The listing builds one solid part. Answer for the finished solid, in the listing's coordinates (mm). A direction names the side the tool comes from. Give positions to 0.01 mm unless a question says otherwise; leave off trailing zeros. Write each loop counter-clockwise with the first axis right and the second up, starting at its lowest first coordinate (ties: lowest second). Pieces come first, ordered by that corner, then holes. Notation, with made-up numbers: (42, 23.5) -> (69, 23.5) arc R18 cw to (69, 49.5) -> close; hole circle Ø3 at (3.5, -33.5). An arc over 180 degrees is marked (long way). One line per question, with ' | ' between items.
Autodesk Inventor part; units mm, degrees
ref_plane "YZ Plane" through (0, 0, 0) normal (1, 0, 0) x (0, 1, 0)
ref_plane "XZ Plane" through (0, 0, 0) normal (0, 1, 0) x (-1, 0, 0)
ref_plane "XY Plane" through (0, 0, 0) normal (0, 0, 1) x (1, 0, 0)
sketch "Esquisse1" plane through (0, 0, 0) normal (0, 1, 0) x (-1, 0, 0)
  line L0 (0, 0) -> (36, 0) construction
  line L1 (36, 0) -> (36, 8) construction
  line L2 (0, 0) -> (0, 13.5) construction
  line L3 (0, 13.5) -> (6.5, 13.5) construction
  line L4 (6.5, 13.5) -> (14.5, 13.5) construction
  line L5 (14.5, 13.5) -> (22.5, 13.5) construction
  line L6 (22.5, 13.5) -> (30.5, 13.5) construction
  circle A0 centre (6.5, 13.5) radius 1
  circle A1 centre (14.5, 13.5) radius 1
  circle A2 centre (22.5, 13.5) radius 1
  circle A3 centre (30.5, 13.5) radius 1
  circle A4 centre (36, 8) radius 1
  circle A5 centre (6.5, -13.5) radius 1
  circle A6 centre (14.5, -13.5) radius 1
  circle A7 centre (22.5, -13.5) radius 1
  circle A8 centre (30.5, -13.5) radius 1
  circle A9 centre (36, -8) radius 1
  line L7 (6.5, 13.5) -> (6.5, 18.5) construction
  line L8 (36, 8) -> (41, 8) construction
  circle A10 centre (0, 0) radius 12 construction
  line L9 (0, 18.5) -> (41, 18.5)
  line L10 (41, 18.5) -> (41, -18.5)
  line L11 (41, -18.5) -> (0, -18.5)
  line L12 (6.5, -13.5) -> (6.5, -18.5) construction
  line L13 (0, 18.5) -> (0, 12)
  line L14 (0, 0) -> (0, -18.5) construction
  line L15 (0, -12) -> (0, -18.5)
  arc A11 (0, -12) -> (0, 12) centre (0, 0) ccw
  dimension "d23" = 36
  dimension "d24" = 8
  dimension "d25" = 13.5
  dimension "d26" = 6.5
  dimension "d27" = 8
  dimension "d28" = 8
  dimension "d29" = 8
  dimension "d30" = 2
  dimension "d31" = 5
  dimension "d33" = 24
extrude "Extrusion2" add sketch "Esquisse1" along normal blind 2
fillet "Congé1" radius 2 1 edges at (0, 1, 12)
fillet "Congé2" radius 2 1 edges at (0, 1, -12)
properties part number "AX12_gabarit"
Item 1: Consider line 1 (Z direction, x = -22.5, y = 0.85); line 2 (Z direction, x = -6.5, y = 1.3); line 3 (X direction, y = 1.45, z = -13). Determine where each line is inside the solid, lowest interval first. Write a range as [from, to].
Answers below:
line 1: [-18.5, -14.5], [-12.5, 12.5], [14.5, 18.5] | line 2: [-18.5, -14.5], [-12.5, -10.09], [10.09, 12.5], [14.5, 18.5] | line 3: [-41, -31.37], [-29.63, -23.37], [-21.63, -15.37], [-13.63, -7.37], [-5.63, -0.19]
Item 2: Determine the mould class of faces 3 (the face through (-0.501, 1.014, -12.532)), 4 (the face through (-41, 1, 0)), 5 (the face through (-20, 1, 18.5)) for opening direction Z: pulls with the +Z half, pulls with the -Z half, needs draft (parallel to the pull), parting line crosses it, or undercut.
Answers below:
face 3: undercut | face 4: needs draft | face 5: pulls with the +Z half
Item 3: A flat-ended cylindrical pin translates along its axis: pin 1 (1.2 mm diameter, centred on x = -6.5, z = -13.5, fed in from +Y). Find the tip coordinate at first contact, or state that the pin passes through.
Answers below:
pin 1: through
Item 4: Find section B-B (y = 1.35). Count the separate pieces of the cut face and the enclosed holes in it, then the cut area to 3 significant figures.
Answers below:
separate pieces: 1 | enclosed holes: 10 | area: 1,260 mm²
Item 5: Find section A-A (x = -14.5). Write down the section's boundary in (y, z), then the cut area to 3 significant figures.
Answers below:
outline: (0, -18.5) -> (2, -18.5) -> (2, -14.5) -> (0, -14.5) -> close; (0, -12.5) -> (2, -12.5) -> (2, 12.5) -> (0, 12.5) -> close; (0, 14.5) -> (2, 14.5) -> (2, 18.5) -> (0, 18.5) -> close | area: 66.0 mm²
Item 6: Find section D-D (x = -6). Write down the section's boundary in (y, z).
Answers below:
outline: (0, -18.5) -> (2, -18.5) -> (2, -14.37) -> (0, -14.37) -> close; (0, -12.63) -> (2, -12.63) -> (2, -10.39) -> (0, -10.39) -> close; (0, 10.39) -> (2, 10.39) -> (2, 12.63) -> (0, 12.63) -> close; (0, 14.37) -> (2, 14.37) -> (2, 18.5) -> (0, 18.5) -> close
Item 7: Find section C-C (z = -8). Write down the section's boundary in (x, y).
Answers below:
outline: (-41, 0) -> (-37, 0) -> (-37, 2) -> (-41, 2) -> close; (-35, 0) -> (-8.94, 0) -> (-8.94, 2) -> (-35, 2) -> close
Item 8: A tool of negligible diameter and unlimited length cuts with its end or side. For faces 1 (the face through (-6.283, 0.986, 14.476)), 2 (the face through (-0.475, 1.014, 12.562)), from which of +Z, -Z, +X, -X, +Y, -Y can it reach the whole face along a straight path? Write none if from no direction.
Answers below:
face 1: +Y, -Y | face 2: +X, +Y, -Y
